Build history of the part. All positions in model axes, mm. Coordinates: 2 decimals unless noted, no trailing zeros. Loops run counter-clockwise (first coordinate to the right, second up) from the corner with the lowest first, then second, coordinate; pieces in that order, holes last. Notation, with made-up numbers: (-15.75, 55.25) - (2.25, 55.25) arc R23 cw to (2.25, 93.25) - close; hole circle Ø5 at (-36.5, 44.25). An arc over 180 degrees is marked (long way). One line per item, written item: value.
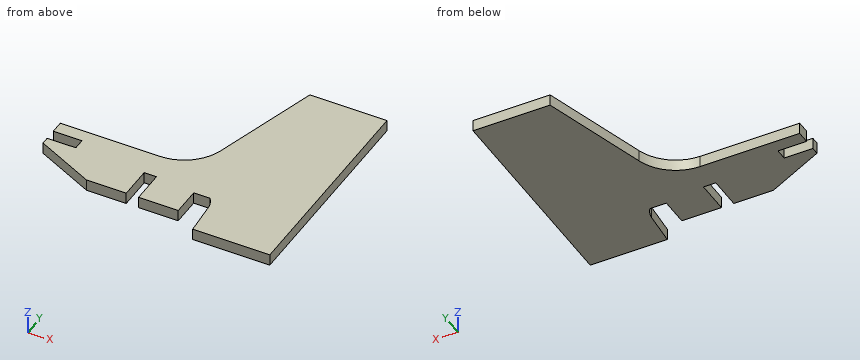
```python
from build123d import *

# Parameters (mm, degrees)
PAD_DEPTH = 2


with BuildPart() as part:
    # CopySketch004 → Pad (new body, symmetric)
    with BuildSketch(Plane.XY):
        with BuildLine():
            Line((-36.508492, 11.060009), (-1.723702, 11.060009))
            ThreePointArc((-1.723702, 11.060009), (7.733856, 14.212769), (13.407871, 22.409771))
            Line((13.407871, 22.409771), (24.319128, 59.832547))
            Line((24.319128, 59.832547), (51.226102, 59.832547))
            Line((51.226102, 59.832547), (51.226102, -16.067453))
            Line((24.319128, -16.067453), (51.226102, -16.067453))
            Line((23.401691, -4.060687), (24.319128, -16.067453))
            ThreePointArc((23.401691, -4.060687), (22.843077, -1.909417), (21.705474, 0))
            Line((16, 0), (21.705474, 0))
            Line((16, -10), (16, 0))
            Line((2.15, -10), (16, -10))
            Line((2.15, 1.647389), (2.15, -10))
            Line((-2.15, 1.647389), (2.15, 1.647389))
            Line((-2.15, -10), (-2.15, 1.647389))
            Line((-16, -10), (-2.15, -10))
            Line((-16, -10), (-36.508492, -0.144815))
            Line((-36.508492, 2.549264), (-36.508492, -0.144815))
            Line((-26.508492, 2.549264), (-36.508492, 2.549264))
            Line((-26.508492, 6.549264), (-26.508492, 2.549264))
            Line((-36.508492, 6.549264), (-26.508492, 6.549264))
            Line((-36.508492, 11.060009), (-36.508492, 6.549264))
        make_face()
    extrude(amount=PAD_DEPTH, both=True)


solid = part.part
```
Item 1: Cut at A-A, the plane z = -0.75. Write the cut outline in (x, y), then the cut area to 3 significant figures.
Check result:
outline: (-36.51, -0.14) - (-16, -10) - (-2.15, -10) - (-2.15, 1.65) - (2.15, 1.65) - (2.15, -10) - (16, -10) - (16, 0) - (21.71, 0) arc R7.87 cw to (23.4, -4.06) - (24.32, -16.07) - (51.23, -16.07) - (51.23, 59.83) - (24.32, 59.83) - (13.41, 22.41) arc R15.76 cw to (-1.72, 11.06) - (-36.51, 11.06) - (-36.51, 6.55) - (-26.51, 6.55) - (-26.51, 2.55) - (-36.51, 2.55) - close
area: 3,430 mm^2
Item 2: Cut at B-B, the plane x = -27.5. Write the cut outline in (y, z), then the cut area to 3 significant figures.
Check result:
outline: (-4.47, -2) - (2.55, -2) - (2.55, 2) - (-4.47, 2) - close; (6.55, -2) - (11.06, -2) - (11.06, 2) - (6.55, 2) - close
area: 46.1 mm^2
Item 3: Probe probe 1 along X at (y, z) = (-6, -0.6); probe 2 along X at (y, z) = (-2, -0.45); probe 3 along Y at (x, z) = (-12, 0.6). List the from-to ranges inside material, lowest first. Write a range as from..to.
Check result:
probe 1: x = -24.32..-2.15, 2.15..16, 23.55..51.23
probe 2: x = -32.65..-2.15, 2.15..16, 22.88..51.23
probe 3: y = -10..11.06
Item 4: Drop flat-ended pins along their axis: P1, Ø1.2, axis at x = -22.5, z = 1, coming from the +Y side; P2, Ø2, axis at x = -6.5, z = 0.5, coming from the -Y side; P3, Ø1.2, axis at x = 19.5, z = -0.5, coming from the -Y side. Give the stop position or say it passes through.
Check result:
P1: stops at y = 11.06
P2: stops at y = -10
P3: stops at y = 0
Item 5: Cut at D-D, the plane y = 3.5. Write the cut outline in (x, z).
Check result:
outline: (-26.51, -2) - (51.23, -2) - (51.23, 2) - (-26.51, 2) - close
Item 6: Cut at C-C, the plane y = -8.5. Write the cut outline in (x, z), then the cut area to 3 significant figures.
Check result:
outline: (-19.12, -2) - (-2.15, -2) - (-2.15, 2) - (-19.12, 2) - close; (2.15, -2) - (16, -2) - (16, 2) - (2.15, 2) - close; (23.74, -2) - (51.23, -2) - (51.23, 2) - (23.74, 2) - close
area: 233 mm^2
